```python
from build123d import *

# Parameters (mm, degrees)
SKETCH1_W                 = 16.51
SKETCH1_H                 = 17.78
BOSS_EXTRUDE1_DEPTH       = 1.6
F_4_CLEARANCE_HOLE1_D     = 2.9464
F_4_CLEARANCE_HOLE1_DEPTH = 6.35
F_4_CLEARANCE_HOLE1_TIP   = 0.885187864
SKETCH4_W                 = 6.4
SKETCH4_H                 = 3
BOSS_EXTRUDE2_DEPTH       = 6.1
SKETCH5_R                 = 0.635
BOSS_EXTRUDE3_DEPTH       = 1.65


with BuildPart() as part:
    # Sketch1 → Boss-Extrude1 (new body)
    with BuildSketch(Plane.XY):
        Rectangle(SKETCH1_W, SKETCH1_H)
    extrude(amount=BOSS_EXTRUDE1_DEPTH)

    # #4 Clearance Hole1
    with Locations(Plane(origin=(0, 6.35, 1.6), x_dir=(1, 0, 0), z_dir=(0, 0, 1))):
        with Locations((0, 0), (0, -12.7)):
            Hole(F_4_CLEARANCE_HOLE1_D / 2, depth=F_4_CLEARANCE_HOLE1_DEPTH)
            with Locations((0, 0, -(F_4_CLEARANCE_HOLE1_DEPTH + F_4_CLEARANCE_HOLE1_TIP / 2))):  # 118° drill point
                Cone(0, F_4_CLEARANCE_HOLE1_D / 2, F_4_CLEARANCE_HOLE1_TIP, mode=Mode.SUBTRACT)

    # Sketch4 → Boss-Extrude2 (add)
    with BuildSketch(Plane.XY.offset(1.6)):
        with Locations((4.19, 0)):
            Rectangle(SKETCH4_W, SKETCH4_H)
    extrude(amount=BOSS_EXTRUDE2_DEPTH)

    # Sketch5 → Boss-Extrude3 (add)
    with BuildSketch(Plane.XY.offset(7.7)):
        with Locations((2.54, 0)):
            Circle(SKETCH5_R)
    extrude(amount=BOSS_EXTRUDE3_DEPTH)


solid = part.part
```
Can you work these out from the model? Positions are in its coordinate system, mm. A direction names the side the tool comes from. Round coordinates to 2 decimals unless told otherwise and drop trailing zeros. Loops run counter-clockwise (first coordinate to the right, second up) from the corner with the lowest first, then second, coordinate; pieces in that order, holes last. Notation, with made-up numbers: M 60.25,5.25 L 67.25,5.25 A20 cw 67.25,9.25 Z; hole C 4,-18 d9. An arc over 180 degrees is marked long. Answer as a JSON object with one key per item and string values. Group by question number.
Q1. Imagine slicing it at B-B, the plane x = 0. Please give me the cut outline in (y, z).
Q2. We'd pull the mould along Y, two halves only. Please class faces 5 (the flat face through (0.99, 0, 5)), 6 (the cylindrical face through (0.19, -4.89, 0.79)), 7 (the flat face through (0, 8.89, 1)), 8 (the cylindrical face through (-0.792, 7.592, 0.789)): +Y half, -Y half, draft (parallel to the pull), parting line (faces both ways), or undercut.
Q3. Imagine slicing it at A-A, the plane y = -6.35. Please give me the cut outline in (x, z) (3 decimals), then the cut area to 3 significant figures.
Q4. Please list where these lines run through material, in increasing order: L1, parallel to Y at x = 0, z = 0.65; L2, parallel to Z at x = 0.5, y = 4; L3, parallel to X at y = -5, z = 1.25 (3 decimals).
Q5. Imagine slicing it at D-D, the plane y = 1. Please give me the cut outline in (x, z) (3 decimals).
Q6. Imagine slicing it at C-C, the plane x = 2.54. Please give me the cut outline in (y, z) (3 decimals).
Q7. Will these pins go through, and if not, where does the flat tip stop? pin 1 (1 mm diameter, centred on y = 0.5, z = 4.5, fed in from -X); pin 2 (8.5 mm diameter, centred on x = -3, y = -4.5, fed in from +Z); pin 3 (3 mm diameter, centred on x = 3.5, z = 3.5, fed in from +Y); pin 4 (1.8 mm diameter, centred on x = 0, y = -6.35, fed in from +Z).
Q8. On a 3-axis mill with a long thin cutter (end or side, diameter ignored), from which of +Z, -Z, +X, -X, +Y, -Y can I reach the whole of each face in a straight line? I mean faces 1 (the flat face through (7.39, 0, 5)), 2 (the cylindrical face through (1.906, 0.028, 8.513)), 3 (the flat face through (4, 1.5, 5)), 4 (the flat face through (4, -1.5, 5)). Say none if no direction works.
Findings:
{
 "1": {"outline": "M -8.89,0 L -7.82,0 L -7.82,1.6 L -8.89,1.6 Z; M -4.88,0 L 4.88,0 L 4.88,1.6 L -4.88,1.6 Z; M 7.82,0 L 8.89,0 L 8.89,1.6 L 7.82,1.6 Z"},
 "2": {"face 5": "draft", "face 6": "undercut", "face 7": "+Y half", "face 8": "undercut"},
 "3": {"outline": "M -8.255,0 L -1.473,0 L -1.473,1.6 L -8.255,1.6 Z; M 1.473,0 L 8.255,0 L 8.255,1.6 L 1.473,1.6 Z", "area": "21.7 mm2"},
 "4": {"L1": "y = -8.89 to -7.82, -4.88 to 4.88, 7.82 to 8.89", "L2": "z = 0 to 1.6", "L3": "x = -8.255 to -0.59, 0.59 to 8.255"},
 "5": {"outline": "M -8.255,0 L 8.255,0 L 8.255,1.6 L 7.39,1.6 L 7.39,7.7 L 0.99,7.7 L 0.99,1.6 L -8.255,1.6 Z"},
 "6": {"outline": "M -8.89,0 L 8.89,0 L 8.89,1.6 L 1.5,1.6 L 1.5,7.7 L 0.635,7.7 L 0.635,9.35 L -0.635,9.35 L -0.635,7.7 L -1.5,7.7 L -1.5,1.6 L -8.89,1.6 Z"},
 "7": {"pin 1": "stops at x = 0.99", "pin 2": "stops at z = 1.6", "pin 3": "stops at y = 1.5", "pin 4": "passes through"},
 "8": {"face 1": "+Z, +X, +Y, -Y", "face 2": "+Z", "face 3": "+Z, +X, -X, +Y", "face 4": "+Z, +X, -X, -Y"}
}
